from build123d import *

# Parameters (mm, degrees)
SKETCH_1_R          = 7
EXTRUDE_1_DEPTH     = 14.5
SKETCH_2_R          = 21
CUT_EXTRUDE_1_DEPTH = 8


with BuildPart() as part:
    # Эскиз1 → Бобышка-Вытянуть1 (new, symmetric)
    with BuildSketch(Plane.XY):
        with BuildLine():
            Line((40.9375, 14.970674459), (1.09375, 17.465786869))
            ThreePointArc((1.09375, 17.465786869), (-17.5, 0), (1.09375, -17.465786869))
            Line((1.09375, -17.465786869), (40.9375, -14.970674459))
            ThreePointArc((40.9375, -14.970674459), (55, 0), (40.9375, 14.970674459))
        make_face()
        with Locations(Location((40, 0, 0), (0, 0, 180))):
            Circle(SKETCH_1_R, mode=Mode.SUBTRACT)
        with BuildLine():
            Line((2.693426411, 10.66515139), (4.201923789, 13.277945491))
            Line((4.201923789, 13.277945491), (9.398076211, 10.277945491))
            Line((9.398076211, 10.277945491), (7.889578833, 7.66515139))
            ThreePointArc((7.889578833, 7.66515139), (-5.5, -9.526279442), (2.693426411, 10.66515139))
        make_face(mode=Mode.SUBTRACT)
    extrude(amount=EXTRUDE_1_DEPTH, both=True)

    # Эскиз2 → Вырез-Вытянуть1 (cut, symmetric)
    with BuildSketch(Plane.XY):
        with Locations((40, 0)):
            Circle(SKETCH_2_R)
    extrude(amount=CUT_EXTRUDE_1_DEPTH, both=True, mode=Mode.SUBTRACT)


solid = part.part
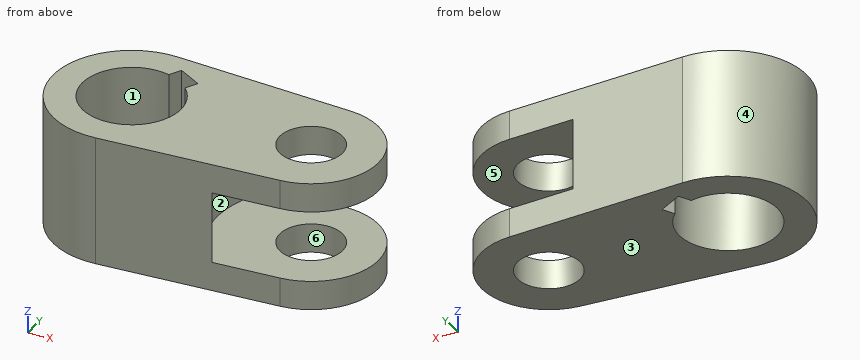
Design review of the part built by this model. Coordinates are the model's own, in mm. Face numbers are marked on the shaded views. A direction names the side the tool comes from. Give positions to 0.01 mm unless a question says otherwise; leave off trailing zeros. Loops run counter-clockwise (first coordinate to the right, second up) from the corner with the lowest first, then second, coordinate; pieces in that order, holes last. Notation, with made-up numbers: (-14.75, 83.5) -> (-10.75, 83.5) arc R27 ccw to (-10.75, 120.5) -> close; hole circle Ø4 at (0, 74). An arc over 180 degrees is marked (long way). One line per question, with ' | ' between items. Start each with the question number.
(1) We need section A-A (z = -12). State the section outline as (x, y) points, and give its area (3 significant figures).
(2) For line 1 (Y direction, x = 0, z = 4.25); line 2 (Z direction, x = 25, y = -0.5); line 3 (X direction, y = -4, z = 2), list the stretches that pass through material, from the lowest coordinate up.
(3) For the marked faces 1 and 2, list the 3-axis set-ups (+Z, -Z, +X, -X, +Y, -Y) from which the entire face can be reached by the end or side of a thin tool; tool diameter is ignored.
(4) We need section C-C (y = -9). State the section outline as (x, z) points.
(5) Insertion check: P1, Ø1.5, axis at y = 13, z = 6, coming from the +X side; P2, Ø12.5, axis at x = 40, y = 0, coming from the -Z side; P3, Ø5, axis at y = 10, z = -0.5, coming from the +X side; P4, Ø2, axis at x = 28.5, z = -10.5, coming from the -Y side. Each pin has a flat end and moves straight along its axis. Give the tip position at first contact, or say it passes through.
(6) Draft analysis for pull direction Y (two halves, no side actions). For the marked faces 3, 4, 5 and 6, state which applies: +Y half, -Y half, draft (parallel to the pull), parting line (faces both ways), or undercut.
(7) We need section B-B (x = 0). State the section outline as (y, z) points, and give its area (3 significant figures).
(8) We need section D-D (x = 38). State the section outline as (y, z) points.
The answers:
1) outline: (1.09, -17.47) -> (40.94, -14.97) arc R15 ccw to (40.94, 14.97) -> (1.09, 17.47) arc R17.5 ccw (long way) to start; hole (2.69, 10.67) arc R11 ccw (long way) to (7.89, 7.67) -> (9.4, 10.28) -> (4.2, 13.28) -> close; hole circle Ø14 at (40, 0) | area: 1,590 mm^2
2) line 1: y = -17.5 to -11, 11 to 17.5 | line 2: z = -14.5 to -8, 8 to 14.5 | line 3: x = -17.04 to -10.25, 10.25 to 19.38
3) face 1: +Z, -Z | face 2: +X
4) outline: (-15.01, -14.5) -> (-6.32, -14.5) -> (-6.32, 14.5) -> (-15.01, 14.5) -> close; (6.32, -14.5) -> (52, -14.5) -> (52, -8) -> (21.03, -8) -> (21.03, 8) -> (52, 8) -> (52, 14.5) -> (6.32, 14.5) -> close
5) P1: stops at x = 24.13 | P2: passes through | P3: stops at x = 23.13 | P4: stops at y = -15.81
6) face 3: draft | face 4: parting line | face 5: undercut | face 6: undercut
7) outline: (-17.5, -14.5) -> (-11, -14.5) -> (-11, 14.5) -> (-17.5, 14.5) -> close; (11, -14.5) -> (17.5, -14.5) -> (17.5, 14.5) -> (11, 14.5) -> close | area: 377 mm^2
8) outline: (-15.15, -14.5) -> (-6.71, -14.5) -> (-6.71, -8) -> (-15.15, -8) -> close; (-15.15, 8) -> (-6.71, 8) -> (-6.71, 14.5) -> (-15.15, 14.5) -> close; (6.71, -14.5) -> (15.15, -14.5) -> (15.15, -8) -> (6.71, -8) -> close; (6.71, 8) -> (15.15, 8) -> (15.15, 14.5) -> (6.71, 14.5) -> close
